The listing builds one solid part. Answer for the finished solid, in the listing's coordinates (mm). Give positions to 0.01 mm unless a question says otherwise; leave off trailing zeros. Loops run counter-clockwise (first coordinate to the right, second up) from the corner with the lowest first, then second, coordinate; pieces in that order, holes last. Notation, with made-up numbers: (89.5, 16.5) - (122.5, 16.5) arc R33 cw to (122.5, 49.5) - close; hole circle Ø1 at (10, 31.25). An arc over 180 degrees is marked (long way). Answer as CSV lines item,"result". Start each with the question number.
1) A cutting plane is placed at A-A (y = 3.6). Determine the outline of the cut face in (x, z) (3 decimals), and give its area (3 significant figures).
2) Flat-ended cylindrical pins translate along their axes: pin 1 (1.7 mm diameter, centred on x = -97, y = 2.5, fed in from +Z); pin 2 (1.7 mm diameter, centred on y = 3.5, z = -76.5, fed in from +X); pin 3 (4 mm diameter, centred on x = -98.42, z = 59.01, fed in from -Y); pin 4 (3 mm diameter, centred on y = 2, z = 77.5, fed in from -X). Find the tip coordinate at first contact, or state that the pin passes through.
3) Find the intervals of material crossed by line 1 along X through (y, z) = (0.3, 73); line 2 along X through (y, z) = (0.85, 60); line 3 along Z through (x, y) = (90.5, 1.5), in increasing order.
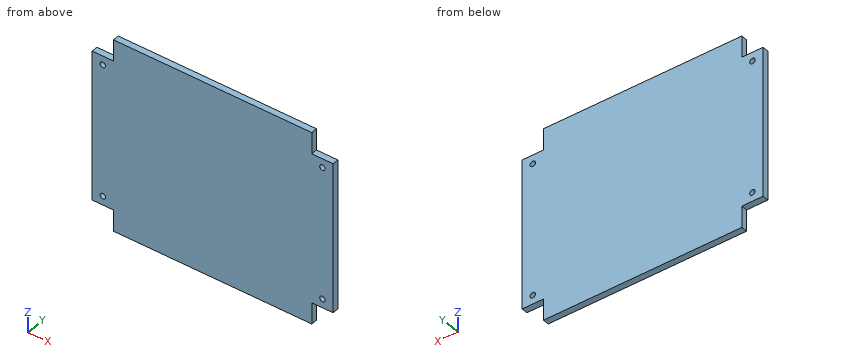
```python
from build123d import *

# Parameters (mm, degrees)
SKETCH1_W           = 215.9
SKETCH1_H           = 172.003199808
BOSS_EXTRUDE1_DEPTH = 5.588
SKETCH2_W           = 19.05
SKETCH2_H           = 19.05
CORNERCUT_DEPTH     = 139.132919429
SKETCH3_R           = 2.4257
MOUNTHOLES_DEPTH    = 139.132919429


with BuildPart() as part:
    # Sketch1 → Boss-Extrude1 (new body)
    with BuildSketch(Plane(origin=(0, 0, 0), x_dir=(1, 0, 0), z_dir=(0, 1, 0))):
        Rectangle(SKETCH1_W, SKETCH1_H)
    extrude(amount=BOSS_EXTRUDE1_DEPTH)

    # Sketch2 → CornerCut (cut, through all)
    with BuildSketch(Plane(origin=(0, 5.588, 0), x_dir=(1, 0, 0), z_dir=(0, 1, 0))):
        with Locations((-98.425, 76.476599904)):
            Rectangle(SKETCH2_W, SKETCH2_H)
        with Locations((98.425, 76.476599904)):
            Rectangle(SKETCH2_W, SKETCH2_H)
        with Locations((98.425, -76.476599904)):
            Rectangle(SKETCH2_W, SKETCH2_H)
        with Locations((-98.425, -76.476599904)):
            Rectangle(SKETCH2_W, SKETCH2_H)
    extrude(amount=-CORNERCUT_DEPTH, mode=Mode.SUBTRACT)

    # Sketch3 → MountHoles (cut, through all)
    with BuildSketch(Plane(origin=(0, 5.588, 0), x_dir=(1, 0, 0), z_dir=(0, 1, 0))):
        with Locations(Location((-98.425, 59.014099904, 0), (0, 0, 270))):
            Circle(SKETCH3_R)
        with Locations(Location((-98.425, -59.014099904, 0), (0, 0, 270))):
            Circle(SKETCH3_R)
        with Locations(Location((98.425, -59.014099904, 0), (0, 0, 270))):
            Circle(SKETCH3_R)
        with Locations(Location((98.425, 59.014099904, 0), (0, 0, 270))):
            Circle(SKETCH3_R)
    extrude(amount=-MOUNTHOLES_DEPTH, mode=Mode.SUBTRACT)


solid = part.part
```
Ans:
1,outline,"(-107.95, -66.952) - (-88.9, -66.952) - (-88.9, -86.002) - (88.9, -86.002) - (88.9, -66.952) - (107.95, -66.952) - (107.95, 66.952) - (88.9, 66.952) - (88.9, 86.002) - (-88.9, 86.002) - (-88.9, 66.952) - (-107.95, 66.952) - close; hole circle Ø4.851 at (-98.425, -59.014); hole circle Ø4.851 at (-98.425, 59.014); hole circle Ø4.851 at (98.425, -59.014); hole circle Ø4.851 at (98.425, 59.014)"
1,area,"35,600 mm2"
2,pin 1,"z = 66.95"
2,pin 2,"x = 88.9"
2,pin 3,"through"
2,pin 4,"x = -88.9"
3,line 1,"-88.9 to 88.9"
3,line 2,"-107.95 to -100.64, -96.21 to 96.21, 100.64 to 107.95"
3,line 3,"-66.95 to 66.95"
